Source: CAD feature listing. Evaluate the final solid. Frame: model axes, mm. A direction names the side the tool comes from. Round coordinates to 2 decimals unless told otherwise and drop trailing zeros. Loops run counter-clockwise (first coordinate to the right, second up) from the corner with the lowest first, then second, coordinate; pieces in that order, holes last.
(1) Set-up query: faces 4 (the cylindrical face through (-0.153, 10.294, 2.325)), 5 (the flat face through (12, 5, 18)), 6 (the flat face through (15, -2, 5)), 7 (the cylindrical face through (0.28, 15.81, 82.6)). Return all of +Z, -Z, +X, -X, +Y, -Y with unobstructed straight access to the full face (end or side cutting, diameter ignored); none if empty.
(2) Section A-A, the plane x = 0. Return the cut outline in (y, z).
(3) Section D-D, the plane z = 68. Return the cut outline in (x, y), plus the area to 3 significant figures.
(4) First-contact query: pin 1 Ø12 at (y, z) = (7.5, 55.5) entering from -X; pin 2 Ø5 at (x, y) = (-16, 10) entering from +Z; pin 3 Ø5.5 at (x, z) = (11, 18.5) entering from +Y; pin 4 Ø2.5 at (y, z) = (0, 15) entering from -X. Flat tips, straight axial feed; report the tip coordinate or a pass-through.
(5) Material intervals for probe 1 along Z at (x, y) = (-10.25, 0); probe 2 along Z at (x, y) = (-5, 7); probe 3 along Z at (x, y) = (17.5, 7), sorted ascending.
(6) Section B-B, the plane z = 5. Return the cut outline in (x, y), plus the area to 3 significant figures.
(7) Mould query, pull axis Z, two halves, no side actions, for faces 1 (the flat face through (0, -12, -5)), 2 (the flat face through (9, 9, 50)), 3 (the cylindrical face through (-0.153, -10.294, 35.21)). Classes: pulls with the +Z half, pulls with the -Z half, needs draft (parallel to the pull), parting line crosses it, or undercut.
(8) Section C-C, the plane y = 7. Return the cut outline in (x, z) (3 decimals).
Autodesk Inventor part; units mm, degrees
ref_plane "YZ Plane" through (0, 0, 0) normal (1, 0, 0) x (0, 1, 0)
ref_plane "XZ Plane" through (0, 0, 0) normal (0, 1, 0) x (-1, 0, 0)
ref_plane "XY Plane" through (0, 0, 0) normal (0, 0, 1) x (1, 0, 0)
ref_plane "Work Plane2" through (0, 0, 20) normal (0, 0, 1) x (1, 0, 0)
sketch "Sketch3" plane through (0, 0, 20) normal (0, 0, 1) x (1, 0, 0)
  line L0 (-11.1369, 5) -> (-11.1369, -5)
  line L1 (-11.1369, 5) -> (-14.9999, 5)
  line L2 (-14.9999, 5) -> (-14.9999, -5)
  line L3 (-14.9999, -5) -> (-11.1369, -5)
  line L4 (-11.1369, -5) -> (-11.1369, 5)
  line L5 (11.1369, 5) -> (14.9999, 5)
  line L6 (14.9999, 5) -> (14.9999, -5)
  line L7 (14.9999, -5) -> (11.1369, -5)
  line L8 (11.1369, -5) -> (11.1369, 5)
  point P0 (0, 0)
  point P1 (0, 0)
  dimension "d9" = 3.863
  dimension "d10" = 3.863
extrude "Extrusion3" add sketch "Sketch3" against normal blind 30
sketch "Sketch4" plane through (-14.9999, -5, 20) normal (-1, 0, 0) x (0, 0, 1)
  line L0 (0, 5) -> (0, 0)
  circle A0 centre (-15, 5) radius 1.5
  circle A1 centre (-5, 5) radius 1.5
  point P0 (-20, 5)
  dimension "d13" = 5
  dimension "d14" = 5
  dimension "d17" = 3
  dimension "d18" = 3
extrude "Extrusion4" cut sketch "Sketch4" against normal blind 200
sketch "Sketch5" plane through (0, 0, 20) normal (0, 0, 1) x (1, 0, 0)
  circle A0 centre (0, 0) radius 20
  circle A1 centre (0, 0) radius 12.2078
  point P0 (-14.9999, 5)
  point P1 (-11.1369, -5)
  point P2 (11.1369, -5)
  point P3 (14.9999, 5)
  dimension "d21" = 40
extrude "Extrusion5" add sketch "Sketch5" along normal blind 30
sketch "Sketch6" plane through (0, 0, 20) normal (0, 0, 1) x (1, 0, 0)
  line L0 (-14.9999, -5) -> (-11.1369, -5)
  line L1 (-14.9999, 5) -> (-11.1369, 5)
  line L2 (-11.1369, -5) -> (-13.4979, -5)
  line L3 (-13.4979, -5) -> (-13.4979, 5)
  line L4 (-13.4979, 5) -> (-11.1369, 5)
  line L5 (-11.1369, 5) -> (-11.1369, -5)
  line L6 (11.1369, -5) -> (11.1369, 5)
  line L7 (11.1369, -5) -> (13.9529, -5)
  line L8 (13.9529, -5) -> (13.9529, 5)
  line L9 (13.9529, 5) -> (11.1369, 5)
  line L10 (11.1369, 5) -> (11.1369, -5)
  arc A0 (11.1369, 5) -> (-11.1369, 5) centre (0, 0) ccw
  arc A1 (-11.1369, -5) -> (11.1369, -5) centre (0, 0) ccw
  arc A2 (-11.1369, 5) -> (-11.1369, -5) centre (0, 0) ccw
  line L11 (14.9999, -5) -> (11.1369, -5)
  line L12 (11.1369, 5) -> (14.9999, 5)
  arc A3 (11.1369, -5) -> (11.1369, 5) centre (0, 0) ccw
extrude "Extrusion6" add sketch "Sketch6" along normal blind 30 contours A2 L5 | L6 A3
sketch "Sketch7" plane through (0, 0, 50) normal (0, 0, 1) x (1, 0, 0)
  line L0 (-14.9999, -5) -> (-11.1369, -5)
  line L1 (-14.9999, 5) -> (-11.1369, 5)
  line L2 (-11.1369, -5) -> (-14.9999, -5)
  line L3 (-14.9999, -5) -> (-14.9999, 5)
  line L4 (-14.9999, 5) -> (-11.1369, 5)
  line L5 (-11.1369, 5) -> (-11.1369, -5)
  arc A0 (-11.1369, -5) -> (11.1369, -5) centre (0, 0) ccw
  line L6 (14.9999, 5) -> (14.9999, -5)
  line L7 (11.1369, -5) -> (14.9999, -5)
  line L8 (14.9999, -5) -> (14.9999, 5)
  line L9 (14.9999, 5) -> (11.1369, 5)
  line L10 (11.1369, 5) -> (11.1369, -5)
extrude "Extrusion7" add sketch "Sketch7" along normal blind 40
sketch "Sketch8" plane through (-14.9999, -5, 50) normal (-1, 0, 0) x (0, 0, 1)
  circle A0 centre (15, 5) radius 1.5
  circle A1 centre (5, 5) radius 1.5
  point P0 (-50, 5)
  point P1 (40, 0)
  dimension "d31" = 3
  dimension "d32" = 3
extrude "Extrusion8" cut sketch "Sketch8" against normal blind 200
sketch "Sketch10" plane through (0, 0, -10) normal (0, 0, -1) x (-1, 0, 0)
  line L0 (11.1369, -5) -> (11.1369, 5)
  line L1 (11.1369, -5) -> (11.9999, -5)
  line L2 (11.9999, -5) -> (11.9999, -3.8424)
  line L3 (11.9999, -3.8424) -> (11.1369, -3.8424)
  line L4 (11.1369, -3.8424) -> (11.1369, -5)
  line L5 (11.9999, -3.8424) -> (11.1369, -3.8424)
  line L6 (11.1369, -3.8424) -> (11.1369, 5)
  line L7 (11.1369, 5) -> (11.9999, 5)
  line L8 (11.9999, 5) -> (11.9999, -3.8424)
  line L9 (-14.9999, -5) -> (-11.1369, -5)
  line L10 (-11.1369, 5) -> (-14.9999, 5)
  line L11 (-11.1369, -5) -> (-11.9999, -5)
  line L12 (-11.9999, -5) -> (-11.9999, 5)
  line L13 (-11.9999, 5) -> (-11.1369, 5)
  line L14 (-11.1369, 5) -> (-11.1369, -5)
  point P0 (0, 0)
  dimension "d35" = 0.863
  dimension "d36" = 0.863
extrude "Extrusion9" cut sketch "Sketch10" against normal blind 200
sketch "Sketch11" plane through (0, 0, 50) normal (0, 0, 1) x (1, 0, 0)
  line L0 (-11.9999, -5) -> (-11.1369, -5)
  line L1 (-11.1369, -5) -> (-11.9999, -5)
  line L2 (-11.9999, -5) -> (-11.9999, 5)
  line L3 (-11.9999, 5) -> (-11.1369, 5)
  line L4 (-11.1369, 5) -> (-11.1369, -5)
  line L5 (11.9999, -5) -> (11.1369, -5)
  line L6 (11.9999, 5) -> (14.9999, 5)
  line L7 (11.1369, -5) -> (11.9999, -5)
  line L8 (11.9999, -5) -> (11.9999, 5)
  line L9 (11.9999, 5) -> (11.1369, 5)
  line L10 (11.1369, 5) -> (11.1369, -5)
  point P0 (0, 0)
extrude "Extrusion10" add sketch "Sketch11" against normal blind 30
sketch "Sketch12" plane through (11.9999, -5, -10) normal (-1, 0, 0) x (0, 0, 1)
  line L0 (100, 10) -> (100, 0)
  line L1 (0, 10) -> (100, 10)
  line L2 (100, 10) -> (100, 0)
  line L3 (100, 0) -> (0, 0)
  line L4 (0, 0) -> (0, 10)
  circle A0 centre (65, 5) radius 1.5
  circle A1 centre (65, 5) radius 1.5
  circle A2 centre (75, 5) radius 1.5
  circle A3 centre (75, 5) radius 1.5
  circle A4 centre (25, 5) radius 1.5
  circle A5 centre (25, 5) radius 1.5
  circle A6 centre (15, 5) radius 1.5
  circle A7 centre (15, 5) radius 1.5
  point P0 (30, 0)
extrude "Extrusion11" add sketch "Sketch12" along normal blind 3
sketch "Sketch13" plane through (-11.9999, -5, -10) normal (1, 0, 0) x (0, 0, -1)
  line L0 (-30, 10) -> (0, 10)
  line L1 (-100, 0) -> (-100, 10)
  line L2 (0, 10) -> (-100, 10)
  line L3 (-100, 10) -> (-100, 0)
  line L4 (-100, 0) -> (0, 0)
  line L5 (0, 0) -> (0, 10)
  circle A0 centre (-65, 5) radius 1.5
  circle A1 centre (-65, 5) radius 1.5
  circle A2 centre (-75, 5) radius 1.5
  circle A3 centre (-75, 5) radius 1.5
  circle A4 centre (-15, 5) radius 1.5
  circle A5 centre (-15, 5) radius 1.5
  circle A6 centre (-25, 5) radius 1.5
  circle A7 centre (-25, 5) radius 1.5
  point P0 (-10, 5)
extrude "Extrusion12" add sketch "Sketch13" along normal blind 3
sketch "Sketch14" plane through (0, 0, -10) normal (0, 0, -1) x (-1, 0, 0)
  line L0 (14.9999, -5) -> (14.9999, 5)
  line L1 (8.9999, -5) -> (8.9999, 5)
  line L2 (8.9999, -5) -> (14.9999, -5)
  line L3 (14.9999, 5) -> (8.9999, 5)
  arc A0 (8.9999, 5) -> (-8.9999, 5) centre (0, 0) ccw
  arc A1 (-8.9999, -5) -> (8.9999, -5) centre (0, 0) ccw
  arc A2 (14.9999, 5) -> (-14.9999, 5) centre (0, 0) ccw
  arc A3 (-14.9999, -5) -> (14.9999, -5) centre (0, 0) ccw
  line L4 (14.9999, 5) -> (8.9999, 5)
  line L5 (-8.9999, 5) -> (-14.9999, 5)
  line L6 (14.9999, -5) -> (8.9999, -5)
  line L7 (-8.9999, -5) -> (-14.9999, -5)
extrude "Extrusion13" add sketch "Sketch14" against normal blind 5
sketch "Sketch19" plane through (0, 0, -5) normal (0, 0, 1) x (1, 0, 0)
  arc A0 (8.9999, 5) -> (-8.9999, 5) centre (0, 0) ccw
  arc A1 (14.9999, 5) -> (-14.9999, 5) centre (0, 0) ccw
  line L0 (14.9999, 5) -> (8.9999, 5)
  line L1 (-8.9999, 5) -> (-14.9999, 5)
  point P0 (8.9999, 5)
extrude "Extrusion17" add sketch "Sketch19" along normal blind 20
sketch "Sketch20" plane through (8.9999, -5, -10) normal (-1, 0, 0) x (0, 0, 1)
  line L0 (100, 10) -> (25, 10)
  line L1 (5, 0) -> (100, 0)
  line L2 (100, 10) -> (90, 10)
  line L3 (90, 10) -> (90, 0)
  line L4 (90, 0) -> (100, 0)
  line L5 (100, 0) -> (100, 10)
  point P0 (10, 5)
  dimension "d62" = 10
extrude "Extrusion18" add sketch "Sketch20" along normal blind 20
sketch "Sketch21" plane through (11.1369, -5, 20) normal (0, -1, 0) x (1, 0, 0)
  line L0 (-20.1369, -5) -> (-20.1369, 60)
  line L1 (-20.1369, 55) -> (-20.1369, 55)
  line L2 (-15.1369, 60) -> (-15.1369, 60)
  line L3 (-2.137, 60) -> (-20.1369, 60)
  line L4 (-2.137, 60) -> (-2.137, -5)
  line L5 (-7.137, 60) -> (-7.137, 60)
  line L6 (-2.137, 55) -> (-2.137, 55)
  arc A0 (-15.1369, 60) -> (-20.1369, 55) centre (-15.1369, 55) ccw
  arc A1 (-2.137, 55) -> (-7.137, 60) centre (-7.137, 55) ccw
  line L7 (-20.1369, 55) -> (-20.1369, 60)
  line L8 (-15.1369, 60) -> (-20.1369, 60)
  line L9 (-7.137, 60) -> (-2.137, 60)
  line L10 (-2.137, 60) -> (-2.137, 55)
  point P0 (-11.1369, -20)
  dimension "d65" = 5
  dimension "d66" = 5
  dimension "d67" = 5
  dimension "d68" = 5
  dimension "d69" = 5
extrude "Extrusion19" add sketch "Sketch21" against normal blind 10
sketch "Sketch22" plane through (0, 0, 50) normal (0, 0, 1) x (1, 0, 0)
  arc A0 (14.9999, 5) -> (-14.9999, 5) centre (0, 0) ccw
  arc A1 (-14.9999, -5) -> (14.9999, -5) centre (0, 0) ccw
  arc A2 (-8.9999, 5) -> (8.9999, 5) centre (0, 0) ccw
  line L0 (14.9999, 5) -> (-14.9999, 5)
  line L1 (-14.9999, 5) -> (14.9999, 5)
  line L2 (-11.1369, -5) -> (-14.9999, -5)
  arc A3 (-14.9999, -5) -> (14.9999, -5) centre (0, 0) ccw
  line L3 (-14.9999, -5) -> (-8.9999, -5)
  line L4 (8.9999, -5) -> (14.9999, -5)
extrude "Extrusion20" add sketch "Sketch22" along normal blind 20 contours L4 A1 L2 L3 A2
sketch "Sketch23" plane through (0, 0, 50) normal (0, 0, -1) x (-1, 0, 0)
  arc A0 (-11.1369, -5) -> (11.1369, -5) centre (0, 0) ccw
  circle A1 centre (0, 0) radius 12.2078
  line L0 (8.9999, 5) -> (8.9999, -5)
  circle A2 centre (0, 0) radius 10.2956
  line L1 (8.9999, -5) -> (11.1369, -5)
  line L2 (-11.1369, 5) -> (-14.9999, 5)
  arc A3 (11.1369, 5) -> (-11.1369, 5) centre (0, 0) ccw
  line L3 (11.1369, -5) -> (8.9999, -5)
  line L4 (-8.9999, -5) -> (-11.1369, -5)
  line L5 (-11.1369, 5) -> (-8.9999, 5)
  line L6 (8.9999, 5) -> (11.1369, 5)
extrude "Extrusion21" add sketch "Sketch23" along normal blind 30 contours L4 A2 L1 A0 | A1 L6 A2 L5
sketch "Sketch24" plane through (-14.9999, 5, 90) normal (0, 1, 0) x (1, 0, 0)
  point P0 (14.9999, 90)
sketch "Sketch25" plane through (0, 0, 90) normal (0, 0, 1) x (1, 0, 0)
  arc A0 (-14.9999, -5) -> (14.9999, -5) centre (0, 0) ccw
  line L0 (-8.9999, 5) -> (-8.9999, -5)
  line L1 (14.9999, 5) -> (-14.9999, 5)
  line L2 (14.9999, 5) -> (-14.9999, 5)
  line L3 (-14.9999, -5) -> (-8.9999, -5)
  line L4 (14.9999, -5) -> (-14.9999, -5)
  arc A1 (-14.9999, -5) -> (14.9999, -5) centre (0, 0) ccw
  arc A2 (14.9999, 5) -> (-14.9999, 5) centre (0, 0) ccw
extrude "Extrusion22" add sketch "Sketch25" against normal blind 15
sketch "Sketch26" plane through (8.9999, 5, 50) normal (0, 1, 0) x (1, 0, 0)
  arc A0 (-5, -30) -> (0, -25) centre (-5, -25) ccw
  line L0 (0, -25) -> (-17.9999, -25)
  line L1 (-12.9999, -30) -> (-5, -30)
  arc A1 (-5, -30) -> (0, -25) centre (-5, -25) ccw
  line L2 (-23.9999, -25) -> (-17.9999, -25)
  arc A2 (-17.9999, -25) -> (-12.9999, -30) centre (-12.9999, -25) ccw
  line L3 (-5, -30) -> (-12.9999, -30)
  point P0 (-8.9999, 50)
extrude "Extrusion23" add sketch "Sketch26" against normal blind 10
sketch "Sketch28" plane through (0, 0, 70) normal (0, 0, 1) x (1, 0, 0)
  line L0 (-14.8626, -5) -> (-8.9999, -5)
  line L1 (8.9999, -5) -> (14.9999, -5)
  line L2 (8.9999, -5) -> (14.9999, -5)
  arc A0 (-14.9999, -5) -> (14.9999, -5) centre (0, 0) ccw
  line L3 (-14.9999, -5) -> (-8.9999, -5)
  line L4 (-14.8626, -5) -> (-14.9999, -5)
  arc A1 (-8.9999, -5) -> (8.9999, -5) centre (0, 0) ccw
  point P0 (0, 0)
extrude "Extrusion24" add sketch "Sketch28" along normal blind 5
properties part number "Part2_abbGripp"
Output values:
1. face 4: -Z
1. face 5: +X, -X, +Y
1. face 6: -Z, +X, +Y, -Y
1. face 7: +Z, +Y
2. outline: (-20, 20) - (-10.3, 20) - (-10.3, 75) - (15.81, 75) - (15.81, 90) - (-15.81, 90) - (-15.81, 50) - (-20, 50) - close; (-15.81, -10) - (-10.3, -10) - (-10.3, -5) - (-15.81, -5) - close; (10.3, -10) - (15.81, -10) - (15.81, 15) - (10.3, 15) - close; (10.3, 20) - (20, 20) - (20, 50) - (10.3, 50) - close
3. outline: (-15, -5) arc R15.81 ccw to (15, -5) - (15, 5) - (9, 5) - (9, -5) arc R10.3 cw to (-9, -5) - (-9, 5) - (-15, 5) - close
3. area: 290 mm2
4. pin 1: stops at x = -19.34
4. pin 2: stops at z = 50
4. pin 3: stops at y = 18.01
4. pin 4: passes through
5. probe 1: z = -10 to 3.5, 6.5 to 13.5, 16.5 to 53.5, 56.5 to 63.5, 66.5 to 90
5. probe 2: z = 75 to 90
5. probe 3: z = 20 to 50
6. outline: (-15, -5) - (-9, -5) - (-9, -1.5) - (-15, -1.5) - close; (-15, 1.5) - (-9, 1.5) - (-9, 5) arc R10.3 cw to (9, 5) - (9, 1.5) - (15, 1.5) - (15, 5) arc R15.81 ccw to (-15, 5) - close; (9, -5) - (15, -5) - (15, -1.5) - (9, -1.5) - close
6. area: 254 mm2
7. face 1: undercut
7. face 2: undercut
7. face 3: needs draft
8. outline: (-18.735, 20) - (-7.55, 20) - (-7.55, 50) - (-18.735, 50) - close; (-14.177, -10) - (-7.55, -10) - (-7.55, 15) - (-14.177, 15) - close; (-14.177, 75) - (14.177, 75) - (14.177, 90) - (-14.177, 90) - close; (7.55, -10) - (14.177, -10) - (14.177, 15) - (7.55, 15) - close; (7.55, 20) - (18.735, 20) - (18.735, 50) - (7.55, 50) - close
